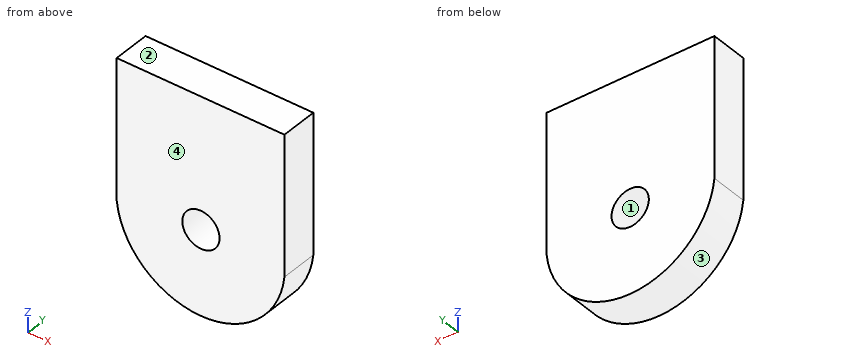
```python
from build123d import *

# Parameters (mm, degrees)
SKETCH330_AS_DRAWN_R                 = 1
EXTRUDE200_DEPTH                     = 5
EXTRUDE200_ONTO_SKETCH330_ROLL_ANGLE = 90
EXTRUDE201_DEPTH                     = 2
EXTRUDE201_ONTO_SKETCH329_ROLL_ANGLE = 90


with BuildPart() as extrude200:
    # Sketch330 as drawn → Extrude200 (new)
    with BuildSketch(Plane.XY):
        with Locations((-45, 11)):
            Circle(SKETCH330_AS_DRAWN_R)
    extrude(amount=-EXTRUDE200_DEPTH)


with BuildPart() as extrude200_1:
    # Extrude200 onto Sketch330 roll: moved
    add(extrude200.part.rotate(Axis((0, 0, 0), (1, 0, 0)), EXTRUDE200_ONTO_SKETCH330_ROLL_ANGLE))


with BuildPart() as extrude200_2:
    # Extrude200 onto Sketch330 placement: moved
    add(extrude200_1.part.moved(Location((0.25, 0, 0))))


with BuildPart() as extrude200_3:
    # Extrude200 placement: moved
    add(extrude200_2.part.moved(Location((0, 8, 0))))


with BuildPart() as obj1:
    # Sketch329 as drawn → Extrude201 (new)
    with BuildSketch(Plane.XY):
        with BuildLine():
            ThreePointArc((-49, 10.52425), (-44.500001, 6.474921), (-40, 10.524249))
            Line((-40, 10.524249), (-40, 18))
            Line((-49, 18), (-40, 18))
            Line((-49, 18), (-49, 10.52425))
        make_face()
    extrude(amount=-EXTRUDE201_DEPTH)


with BuildPart() as obj1_1:
    # Extrude201 onto Sketch329 roll: moved
    add(obj1.part.rotate(Axis((0, 0, 0), (1, 0, 0)), EXTRUDE201_ONTO_SKETCH329_ROLL_ANGLE))


with BuildPart() as obj1_2:
    # Extrude201 onto Sketch329 placement: moved
    add(obj1_1.part)


with BuildPart() as obj1_3:
    # Extrude201 placement: moved
    add(obj1_2.part.moved(Location((-0.27, 10, 0))))

    # Cut107: cut Extrude200
    add(extrude200_3.part, mode=Mode.SUBTRACT)


with BuildPart() as obj1_4:
    # Cut107 placement: moved
    add(obj1_3.part.moved(Location((0, -22, 0))))


solid = obj1_4.part
```
Could you check a few things on this model? Use its own coordinates, in mm. Face numbers are marked on the shaded views. Give positions to 0.01 mm unless a question says otherwise; leave off trailing zeros. Write each loop counter-clockwise with the first axis right and the second up, starting at its lowest first coordinate (ties: lowest second). Pieces come first, ordered by that corner, then holes. Notation, with made-up numbers: (82.5, 35.25) - (92.5, 35.25) arc R20 cw to (92.5, 68.25) - close; hole circle Ø9 at (-35, 58.25). An arc over 180 degrees is marked (long way). One line per item, written item: value. Start each with the question number.
Item 1: Please list where these lines run through material, in increasing order: line 1 (Z direction, x = -44.75, y = -11.1); line 2 (Z direction, x = -44, y = -10.25); line 3 (X direction, y = -10.8, z = 11.5). Write a range as from..to.
Item 2: Imagine slicing it at D-D, the plane x = -43. List the corners of the cut face in (y, z) for me, and give its area (3 significant figures).
Item 3: Imagine slicing it at B-B, the plane z = 11. List the corners of the cut face in (x, y) for me, and give its area (3 significant figures).
Item 4: Imagine slicing it at C-C, the plane x = -44.75. List the corners of the cut face in (y, z) for me, and give its area (3 significant figures).
Item 5: Imagine slicing it at A-A, the plane y = -11.6. List the corners of the cut face in (x, z) for me.
Item 6: If we mould it in two halves opening along Z, with no side actions, what happens to the marked faces 1, 2, 3 and 4? For each: +Z half, -Z half, draft (parallel to the pull), parting line (faces both ways), or undercut.
Geometry says:
1. line 1: 6.47..10, 12..18
1. line 2: 6.54..10.34, 11.66..18
1. line 3: -49.27..-45.62, -43.88..-40.27
2. outline: (-12, 6.84) - (-10, 6.84) - (-10, 18) - (-12, 18) - close
2. area: 22.3 mm^2
3. outline: (-49.27, -12) - (-45.75, -12) - (-45.75, -10) - (-49.27, -10) - close; (-43.75, -12) - (-40.27, -12) - (-40.27, -10) - (-43.75, -10) - close
3. area: 14.0 mm^2
4. outline: (-12, 6.47) - (-10, 6.47) - (-10, 10) - (-12, 10) - close; (-12, 12) - (-10, 12) - (-10, 18) - (-12, 18) - close
4. area: 19.1 mm^2
5. outline: (-49.27, 10.52) arc R4.53 ccw to (-40.27, 10.52) - (-40.27, 18) - (-49.27, 18) - close; hole circle Ø2 at (-44.75, 11)
6. face 1: undercut
6. face 2: +Z half
6. face 3: -Z half
6. face 4: draft
